from build123d import *

# Parameters (mm, degrees)
PAD004_DEPTH    = 8.2
SKETCH014_W     = 28.5
SKETCH014_H     = 6.2
PAD005_DEPTH    = 1.8
SKETCH015_R     = 2.9
POCKET004_DEPTH = 0.6
SKETCH016_W     = 2.05
SKETCH016_H     = 6.2
POCKET005_DEPTH = 1.8


with BuildPart() as part:
    # Sketch013 → Pad004 (new body)
    with BuildSketch(Plane.XY):
        with BuildLine():
            Line((0, 0), (28.5, 0))
            Line((28.5, 0), (28.5, 22.75))
            Line((28.5, 22.75), (14, 22.75))
            Line((14, 22.75), (14, 22.5))
            ThreePointArc((11, 19.5), (13.12132, 20.37868), (14, 22.5))
            Line((11, 19.5), (0, 19.5))
            Line((0, 19.5), (0, 0))
        make_face()
    extrude(amount=PAD004_DEPTH)

    # Sketch014 (on Face9 of Pad004) → Pad005 (join)
    with BuildSketch(Plane.XY.offset(8.2)):
        with Locations((14.25, 9.75)):
            Rectangle(SKETCH014_W, SKETCH014_H)
    extrude(amount=PAD005_DEPTH)

    # Sketch015 (on Face11 of Pad005) → Pocket004 (cut)
    with BuildSketch(Plane.XY.offset(10)):
        with Locations((8.735056, 9.75)):
            Circle(SKETCH015_R)
    extrude(amount=-POCKET004_DEPTH, mode=Mode.SUBTRACT)

    # Sketch016 (on Face10 of Pocket004) → Pocket005 (cut)
    with BuildSketch(Plane.XY.offset(10)):
        with Locations((15.5, 9.75)):
            Rectangle(SKETCH016_W, SKETCH016_H)
        Polygon((21.525, 12.85), (21.525, 6.65), (19.475, 6.65), (19.475, 12.85), (20.5, 12.85), align=None)
        with Locations((25.5, 9.75)):
            Rectangle(SKETCH016_W, SKETCH016_H)
    extrude(amount=-POCKET005_DEPTH, mode=Mode.SUBTRACT)


solid = part.part
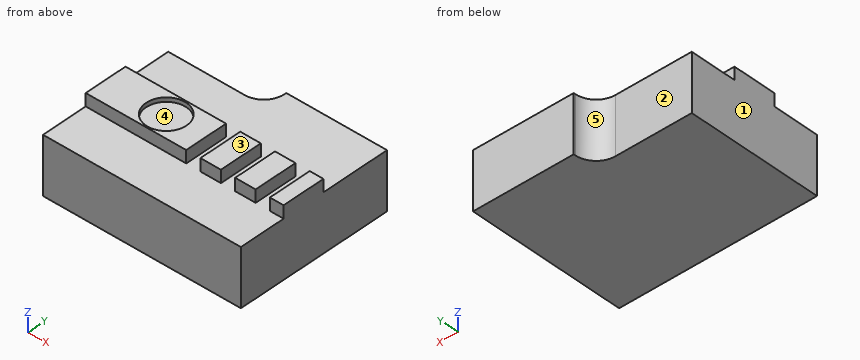
For this review, take the finished solid that the model builds, in its own axes (mm). Face numbers are marked on the shaded views. A direction names the side the tool comes from. Give positions to 0.01 mm unless a question says otherwise; leave off trailing zeros. Loops run counter-clockwise (first coordinate to the right, second up) from the corner with the lowest first, then second, coordinate; pieces in that order, holes last. Notation, with made-up numbers: M 31,-20 L 67,-20 A18 ccw 67,-12 Z; hole C 9,26 d11. An arc over 180 degrees is marked long. Answer as a JSON object with one key per item and string values. Group by question number.
Q1. Add section A-A on y = 9.75. Give the boundary of the cut face in (x, z) (3 decimals), and give its area (3 significant figures).
Q2. Add section B-B on z = 5. Give the boundary of the cut face in (x, y).
Q3. Add section D-D on x = 10.5. Give the boundary of the cut face in (y, z).
Q4. For probe 1 along X at (y, z) = (10, 8.5) (3 decimals); probe 2 along Y at (x, z) = (1, 6.25); probe 3 along Y at (x, z) = (7.5, 9.25), list the stretches that pass through material, from the lowest coordinate up. Write a range as [from, to].
Q5. Add section C-C on x = 2.5. Give the boundary of the cut face in (y, z).
Q6. Mouldability with a two-part tool opening along X and no side actions: class the marked faces 3, 4 and 5 as +X half, -X half, draft (parallel to the pull), parting line (faces both ways), or undercut.
Q7. Tool access review of the marked faces 1 and 2: name each direction out of +Z, -Z, +X, -X, +Y, -Y from which nothing blocks a thin tool from reaching the whole face with its end or side.
Q8. Insertion check: P1, Ø6, axis at x = 5.5, z = 3, coming from the +Y side; P2, Ø0.5, axis at x = 28, z = 9, coming from the -Y side; P3, Ø3, axis at x = 10.5, z = 7.5, coming from the +Y side. Each pin has a flat end and moves straight along its axis. Give the tip position at first contact, or say it passes through.
Checked values:
{
 "1": {"outline": "M 0,0 L 28.5,0 L 28.5,10 L 26.525,10 L 26.525,8.2 L 24.475,8.2 L 24.475,10 L 21.525,10 L 21.525,8.2 L 19.475,8.2 L 19.475,10 L 16.525,10 L 16.525,8.2 L 14.475,8.2 L 14.475,10 L 11.635,10 L 11.635,9.4 L 5.835,9.4 L 5.835,10 L 0,10 Z", "area": "270 mm²"},
 "2": {"outline": "M 0,0 L 28.5,0 L 28.5,22.75 L 14,22.75 L 14,22.5 A3 cw 11,19.5 L 0,19.5 Z"},
 "3": {"outline": "M 0,0 L 19.5,0 L 19.5,8.2 L 12.85,8.2 L 12.85,10 L 12.05,10 L 12.05,9.4 L 7.45,9.4 L 7.45,10 L 6.65,10 L 6.65,8.2 L 0,8.2 Z"},
 "4": {"probe 1": "[0, 14.475], [16.525, 19.475], [21.525, 24.475], [26.525, 28.5]", "probe 2": "[0, 19.5]", "probe 3": "[6.65, 12.85]"},
 "5": {"outline": "M 0,0 L 19.5,0 L 19.5,8.2 L 12.85,8.2 L 12.85,10 L 6.65,10 L 6.65,8.2 L 0,8.2 Z"},
 "6": {"face 3": "draft", "face 4": "undercut", "face 5": "-X half"},
 "7": {"face 1": "+Z, -Z, -X, +Y, -Y", "face 2": "+Z, -Z, -X, +Y"},
 "8": {"P1": "y = 19.5", "P2": "y = 6.65", "P3": "y = 19.67"}
}
